Study the drawing (mm; zero at the part's minimum x, y, z) and answer. A direction names the side the tool comes from. Round coordinates to 2 decimals unless told otherwise and drop trailing zeros. Loops run counter-clockwise (first coordinate to the right, second up) from the corner with the lowest first, then second, coordinate; pieces in that order, holes last. Notation, with made-up numbers: M 35.5,10.5 L 81.5,10.5 A18 cw 81.5,40.5 Z; hole C -15.75,-2 d5. An arc over 180 degrees is marked long. Write each question's results on one line, items separated by ' | '.
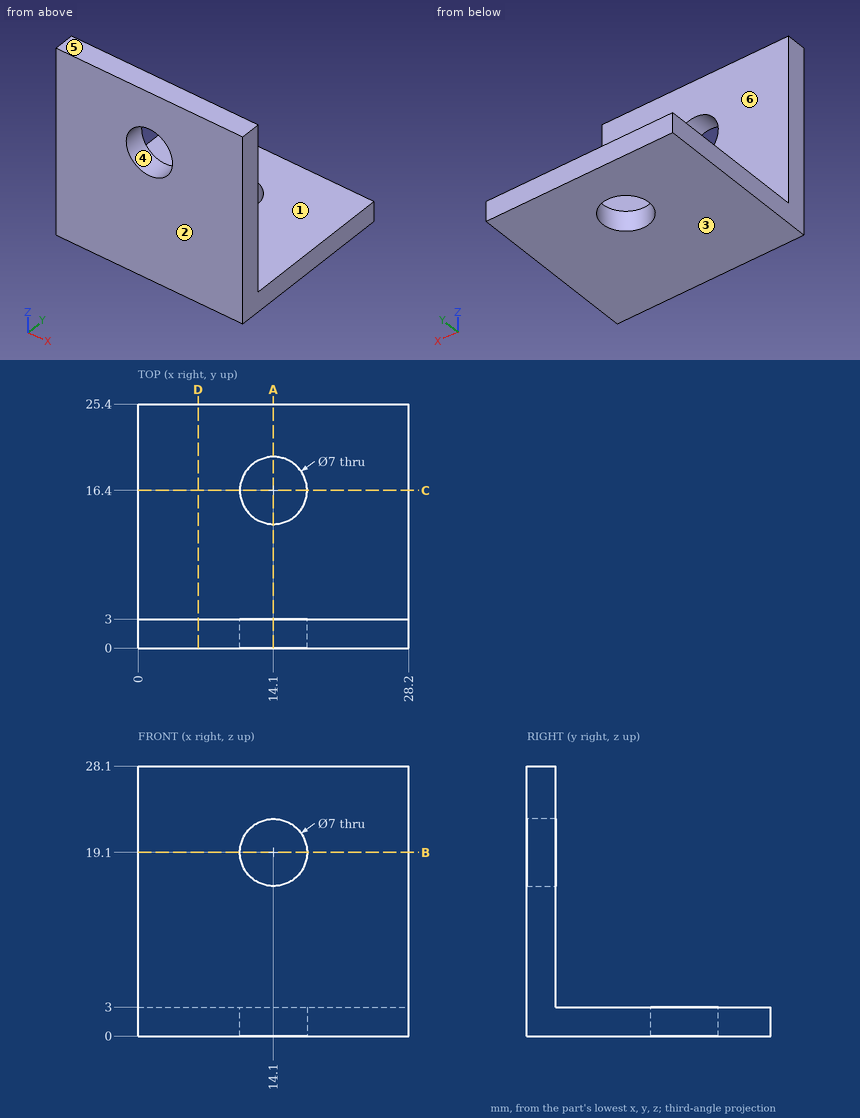
Item 1: The mould has two halves that part along Z. Classify the marked faces 3, 4, 5 and 6: pulls with the +Z half, pulls with the -Z half, needs draft (parallel to the pull), parting line crosses it, or undercut.
Outcome:
face 3: pulls with the -Z half | face 4: undercut | face 5: pulls with the +Z half | face 6: needs draft
Item 2: Flat-ended cylindrical pins translate along their axes: pin 1 (2 mm diameter, centred on x = 7, z = 11, fed in from +Y); pin 2 (3 mm diameter, centred on x = 9, z = 19, fed in from -Y). Find the tip coordinate at first contact, or state that the pin passes through.
Outcome:
pin 1: stops at y = 3 | pin 2: stops at y = 0
Item 3: Straight lines are drawn through the part: line 1 (Y direction, x = 14.1, z = 1.25); line 2 (Y direction, x = 9, z = 26.25); line 3 (X direction, y = 2.2, z = 19.1). For each, find the intervals that lie inside material, in ascending order.
Outcome:
line 1: y = 0 to 12.9, 19.9 to 25.4 | line 2: y = 0 to 3 | line 3: x = 0 to 10.6, 17.6 to 28.2
Item 4: The part is cut by section B-B (z = 19.1). Determine the outline of the cut face in (x, y), plus the area to 3 significant figures.
Outcome:
outline: M 0,0 L 10.6,0 L 10.6,3 L 0,3 Z; M 17.6,0 L 28.2,0 L 28.2,3 L 17.6,3 Z | area: 63.6 mm2
Item 5: For the marked faces 1 and 2, determine the directions among +Z, -Z, +X, -X, +Y, -Y from which every point of the face is accessible in a straight line to the end or side of a thin tool.
Outcome:
face 1: +Z, +X, -X, +Y | face 2: +Z, -Z, +X, -X, -Y
Item 6: The part is cut by section A-A (x = 14.1). Determine the outline of the cut face in (y, z).
Outcome:
outline: M 0,0 L 12.9,0 L 12.9,3 L 3,3 L 3,15.6 L 0,15.6 Z; M 0,22.6 L 3,22.6 L 3,28.1 L 0,28.1 Z; M 19.9,0 L 25.4,0 L 25.4,3 L 19.9,3 Z
Item 7: The part is cut by section D-D (x = 6.25). Determine the outline of the cut face in (y, z).
Outcome:
outline: M 0,0 L 25.4,0 L 25.4,3 L 3,3 L 3,28.1 L 0,28.1 Z
